Autodesk Inventor part; units mm, degrees
ref_plane "Work Plane1" through (0, 42.672, 0) normal (0, 1, 0) x (1, 0, 0)
ref_plane "YZ Plane" through (0, 0, 0) normal (1, 0, 0) x (0, 1, 0)
ref_plane "XZ Plane" through (0, 0, 0) normal (0, 1, 0) x (-1, 0, 0)
sketch "Sketch1" plane through (0, 0, 0) normal (0, 1, 0) x (-1, 0, 0)
  line L0 (-11.1125, 29.21) -> (11.1125, 29.21)
  line L1 (14.2875, 26.035) -> (14.2875, -26.035)
  line L2 (11.1125, -29.21) -> (-11.1125, -29.21)
  line L3 (-14.2875, -26.035) -> (-14.2875, 26.035)
  line L4 (-14.2875, 29.21) -> (14.2875, -29.21) construction
  line L5 (14.2875, 29.21) -> (-14.2875, -29.21) construction
  arc A0 (14.2875, 26.035) -> (11.1125, 29.21) centre (11.1125, 26.035) ccw
  arc A1 (-11.1125, 29.21) -> (-14.2875, 26.035) centre (-11.1125, 26.035) ccw
  arc A2 (-14.2875, -26.035) -> (-11.1125, -29.21) centre (-11.1125, -26.035) ccw
  arc A3 (11.1125, -29.21) -> (14.2875, -26.035) centre (11.1125, -26.035) ccw
  point P0 (0, 0)
  dimension "d0" = 28.575
  dimension "d1" = 58.42
  dimension "d2" = 3.175
extrude "Extrusion1" add sketch "Sketch1" along normal blind 46.482
ref_plane "Work Plane1" through (0, 42.672, 0) normal (0, 1, 0) x (1, 0, 0)
sketch "Sketch2" plane through (0, 42.672, 0) normal (0, 1, 0) x (1, 0, 0)
  arc A0 (-11.1125, 29.21) -> (-14.2875, 26.035) centre (-11.1125, 26.035) ccw
  line L0 (-11.1125, 29.21) -> (11.1125, 29.21)
  arc A1 (14.2875, 26.035) -> (11.1125, 29.21) centre (11.1125, 26.035) ccw
  line L1 (14.2875, 26.035) -> (14.2875, -26.035)
  arc A2 (11.1125, -29.21) -> (14.2875, -26.035) centre (11.1125, -26.035) ccw
  line L2 (11.1125, -29.21) -> (-11.1125, -29.21)
  arc A3 (-14.2875, -26.035) -> (-11.1125, -29.21) centre (-11.1125, -26.035) ccw
  line L3 (-14.2875, -26.035) -> (-14.2875, 26.035)
  line L4 (-11.1125, -36.8935) -> (11.1125, -36.8935)
  line L5 (14.2875, -33.7185) -> (14.2875, 33.7185)
  line L6 (11.1125, 36.8935) -> (-6.604, 36.8935)
  line L7 (-14.2875, 33.7185) -> (-14.2875, -33.7185)
  line L8 (-14.2875, -36.8935) -> (14.2875, 36.8935) construction
  line L9 (14.2875, -36.8935) -> (-14.2875, 36.8935) construction
  arc A4 (-11.1125, 36.8935) -> (-14.2875, 33.7185) centre (-11.1125, 33.7185) ccw
  arc A5 (14.2875, 33.7185) -> (11.1125, 36.8935) centre (11.1125, 33.7185) ccw
  arc A6 (11.1125, -36.8935) -> (14.2875, -33.7185) centre (11.1125, -33.7185) ccw
  arc A7 (-14.2875, -33.7185) -> (-11.1125, -36.8935) centre (-11.1125, -33.7185) ccw
  line L10 (-7.874, -33.655) -> (7.874, -33.655) construction
  line L11 (7.874, -33.655) -> (7.874, 33.655) construction
  line L12 (7.874, 33.655) -> (-7.874, 33.655) construction
  line L13 (-7.874, 33.655) -> (-7.874, -33.655) construction
  line L14 (-7.874, -33.655) -> (7.874, 33.655) construction
  line L15 (7.874, -33.655) -> (-7.874, 33.655) construction
  arc A8 (-9.144, 35.0749) -> (-6.604, 35.0749) centre (-7.874, 33.655) ccw
  line L16 (-9.144, 32.385) -> (-6.604, 32.385) construction
  line L17 (-6.604, 32.385) -> (-6.604, 34.925) construction
  line L18 (-6.604, 34.925) -> (-9.144, 34.925) construction
  line L19 (-9.144, 34.925) -> (-9.144, 32.385) construction
  line L20 (-9.144, 32.385) -> (-6.604, 34.925) construction
  line L21 (-6.604, 32.385) -> (-9.144, 34.925) construction
  line L22 (-9.144, 34.925) -> (-6.604, 34.925) construction
  line L23 (-6.604, 34.925) -> (-6.604, 36.8935)
  line L24 (-6.604, 36.8935) -> (-9.144, 36.8935)
  line L25 (-9.144, 36.8935) -> (-9.144, 34.925)
  arc A9 (-6.604, 35.0749) -> (-9.144, 35.0749) centre (-7.874, 33.655) ccw construction
  line L26 (-9.144, 36.8935) -> (-11.1125, 36.8935)
  line L27 (-6.604, 36.8935) -> (-9.144, 36.8935) construction
  arc A10 (6.604, 35.0749) -> (9.144, 35.0749) centre (7.874, 33.655) ccw
  line L28 (6.604, 36.8935) -> (6.604, 34.925)
  line L29 (9.144, 34.925) -> (9.144, 36.8935)
  line L30 (-14.2875, 0) -> (14.2875, 0) construction
  arc A11 (-6.604, -35.0749) -> (-9.144, -35.0749) centre (-7.874, -33.655) ccw
  line L31 (-6.604, -34.925) -> (-6.604, -36.8935)
  line L32 (-9.144, -36.8935) -> (-9.144, -34.925)
  arc A12 (9.144, -35.0749) -> (6.604, -35.0749) centre (7.874, -33.655) ccw
  line L33 (6.604, -36.8935) -> (6.604, -34.925)
  line L34 (9.144, -34.925) -> (9.144, -36.8935)
  line L35 (6.604, 36.8935) -> (9.144, 36.8935) construction
  line L36 (6.604, -36.8935) -> (9.144, -36.8935) construction
  line L37 (-9.144, -36.8935) -> (-6.604, -36.8935) construction
  line L38 (6.604, 36.8935) -> (9.144, 36.8935)
  line L39 (6.604, -36.8935) -> (9.144, -36.8935)
  line L40 (-9.144, -36.8935) -> (-6.604, -36.8935)
  point P0 (0, 0)
  dimension "d6" = 73.787
  dimension "d7" = 3.175
  dimension "d10" = 15.748
  dimension "d11" = 67.31
  dimension "d12" = 3.81
  dimension "d16" = 2.54
  dimension "d17" = 2.54
  dimension "d20" = 15.748
extrude "Extrusion2" add sketch "Sketch2" against normal blind 3.81 contours A0 L7 A4 L26 L25 A8 L23 L6 L28 A10 L29 A5 L5 A1 L0 | A3 L2 A2 L5 A6 L4 L34 A12 L33 L31 A11 L32 A7 L7 | L24 L23 A8 L25 | L32 A11 L31 L4 | L29 A10 L28 L6 | L4 L33 A12 L34
extrude "Extrusion3" cut sketch "Sketch2" against normal through all contours L24 L23 A8 L25 | L32 A11 L31 L4 | L29 A10 L28 L6 | L4 L33 A12 L34
sketch "Sketch3" plane through (0, 46.482, 0) normal (0, 1, 0) x (1, 0, 0)
  line L0 (-14.2875, 26.035) -> (-14.2875, -26.035) construction
  arc A0 (-14.2875, -26.035) -> (-11.1125, -29.21) centre (-11.1125, -26.035) ccw construction
  line L1 (-11.1125, -29.21) -> (11.1125, -29.21) construction
  arc A1 (11.1125, -29.21) -> (14.2875, -26.035) centre (11.1125, -26.035) ccw construction
  line L2 (14.2875, -26.035) -> (14.2875, 26.035) construction
  arc A2 (14.2875, 26.035) -> (11.1125, 29.21) centre (11.1125, 26.035) ccw construction
  line L3 (11.1125, 29.21) -> (-11.1125, 29.21) construction
  arc A3 (-11.1125, 29.21) -> (-14.2875, 26.035) centre (-11.1125, 26.035) ccw construction
  circle A4 centre (0, 14.9225) radius 14.2875
  line L4 (-13.3985, -18.034) -> (-13.3985, 9.9614)
  line L5 (13.3985, -18.034) -> (13.3985, 9.9614)
  line L6 (-13.3985, -18.034) -> (13.3985, -18.034)
  circle A5 centre (0, -18.034) radius 6.35 construction
  line L7 (0, -18.034) -> (0, -21.844) construction
  arc A6 (-6.35, -18.034) -> (6.35, -18.034) centre (0, -14.6473) ccw
  point P0 (0, 0)
  dimension "d27" = 0.889
  dimension "d28" = 0.889
  dimension "d29" = 47.244
  dimension "d30" = 12.7
  dimension "d31" = 3.81
extrude "Extrusion4" add sketch "Sketch3" along normal blind 3.81
sketch "Sketch4" plane through (0, 50.292, 0) normal (0, 1, 0) x (1, 0, 0)
  arc A0 (13.3985, 9.9614) -> (-13.3985, 9.9614) centre (0, 14.9225) ccw construction
  circle A1 centre (0, 14.9225) radius 6.9215
  point P0 (0, 0)
  dimension "d34" = 13.843
extrude "Extrusion5" add sketch "Sketch4" along normal blind 2.54
sketch "Sketch5" plane through (0, 50.292, 0) normal (0, 1, 0) x (1, 0, 0)
  circle A0 centre (0, 14.9225) radius 6.9215 construction
  arc A1 (-6.35, -18.034) -> (6.35, -18.034) centre (0, -14.6473) ccw construction
  line L0 (6.35, -18.034) -> (13.3985, -18.034) construction
  line L1 (13.3985, -18.034) -> (13.3985, 9.9614) construction
  arc A2 (13.3985, 9.9614) -> (-13.3985, 9.9614) centre (0, 14.9225) ccw construction
  line L2 (-13.3985, 9.9614) -> (-13.3985, -18.034) construction
  line L3 (-13.3985, -18.034) -> (-6.35, -18.034) construction
  line L4 (-9.906, -2.159) -> (9.9036, -2.159) construction
  line L5 (9.9036, -2.159) -> (9.9036, -14.859) construction
  line L6 (9.9036, -14.859) -> (-9.906, -14.859) construction
  line L7 (-9.906, -14.859) -> (-9.906, -2.159) construction
  point P0 (0, 0)
  dimension "d53" = 12.7
  dimension "d59" = 3.175
  dimension "d60" = 3.4925
  dimension "d61" = 3.4949
decal "Decal1"
sketch "Sketch6" plane through (0, 52.832, -14.9225) normal (0, 1, 0) x (1, 0, 0)
  circle A0 centre (0, 0) radius 6.9215 construction
  circle A1 centre (0, 0) radius 2.8575
  point P0 (0, -14.9225)
  dimension "d62" = 5.715
extrude "Extrusion6" add sketch "Sketch6" along normal blind 3.175
hole "Hole1" at (0, 56.007, -14.9225) direction (0, -1, 0) diameter 2.54 depth 25.4 tip angle 118 countersink diameter 3.81 countersink angle 82
sketch "Sketch7" plane through (0, 0, 0) normal (0, -1, 0) x (1, 0, 0)
  line L0 (-14.2875, 26.035) -> (-14.2875, -26.035) construction
  arc A0 (-14.2875, -26.035) -> (-11.1125, -29.21) centre (-11.1125, -26.035) ccw construction
  line L1 (-11.1125, -29.21) -> (11.1125, -29.21) construction
  arc A1 (11.1125, -29.21) -> (14.2875, -26.035) centre (11.1125, -26.035) ccw construction
  line L2 (14.2875, -26.035) -> (14.2875, 26.035) construction
  arc A2 (14.2875, 26.035) -> (11.1125, 29.21) centre (11.1125, 26.035) ccw construction
  line L3 (11.1125, 29.21) -> (-11.1125, 29.21) construction
  arc A3 (-11.1125, 29.21) -> (-14.2875, 26.035) centre (-11.1125, 26.035) ccw construction
  line L4 (-14.2875, 26.035) -> (-14.2875, 33.7185) construction
  line L5 (14.2875, -26.035) -> (14.2875, -33.7185) construction
  line L6 (-14.2875, 29.21) -> (14.2875, 29.21) construction
  line L7 (14.2875, 29.21) -> (14.2875, -29.21) construction
  line L8 (14.2875, -29.21) -> (-14.2875, -29.21) construction
  line L9 (-14.2875, -29.21) -> (-14.2875, 29.21) construction
  line L10 (-11.1125, 22.86) -> (-14.2875, 22.86)
  line L11 (-14.2875, 22.86) -> (-14.2875, 29.21)
  line L12 (-14.2875, 29.21) -> (-7.9375, 29.21)
  line L13 (-7.9375, 29.21) -> (-7.9375, 26.035)
  line L14 (-7.9375, 22.86) -> (-14.2875, 29.21) construction
  line L15 (-14.2875, 22.86) -> (-7.9375, 29.21) construction
  line L16 (11.1125, 22.86) -> (14.2875, 22.86)
  line L17 (14.2875, 22.86) -> (14.2875, 29.21)
  line L18 (14.2875, 29.21) -> (7.9375, 29.21)
  line L19 (7.9375, 29.21) -> (7.9375, 26.035)
  line L20 (7.9375, 22.86) -> (14.2875, 29.21) construction
  line L21 (14.2875, 22.86) -> (7.9375, 29.21) construction
  line L22 (-11.1125, -22.86) -> (-14.2875, -22.86)
  line L23 (-14.2875, -22.86) -> (-14.2875, -29.21)
  line L24 (-14.2875, -29.21) -> (-7.9375, -29.21)
  line L25 (-7.9375, -29.21) -> (-7.9375, -26.035)
  line L26 (-7.9375, -22.86) -> (-14.2875, -29.21) construction
  line L27 (-14.2875, -22.86) -> (-7.9375, -29.21) construction
  line L28 (11.1125, -22.86) -> (14.2875, -22.86)
  line L29 (14.2875, -22.86) -> (14.2875, -29.21)
  line L30 (14.2875, -29.21) -> (7.9375, -29.21)
  line L31 (7.9375, -29.21) -> (7.9375, -26.035)
  line L32 (7.9375, -22.86) -> (14.2875, -29.21) construction
  line L33 (14.2875, -22.86) -> (7.9375, -29.21) construction
  arc A4 (-11.1125, 22.86) -> (-7.9375, 26.035) centre (-11.1125, 26.035) ccw
  arc A5 (7.9375, 26.035) -> (11.1125, 22.86) centre (11.1125, 26.035) ccw
  arc A6 (-7.9375, -26.035) -> (-11.1125, -22.86) centre (-11.1125, -26.035) ccw
  arc A7 (11.1125, -22.86) -> (7.9375, -26.035) centre (11.1125, -26.035) ccw
  point P0 (0, 0)
  dimension "d76" = 3.175
extrude "Extrusion7" cut sketch "Sketch7" against normal blind 1.27
properties part number "HS-785HB-1111-2017" material "Plastic, Opaque Black"
For this review, take the finished solid that the model builds, in its own axes (mm). A direction names the side the tool comes from. Give positions to 0.01 mm unless a question says otherwise; leave off trailing zeros. Loops run counter-clockwise (first coordinate to the right, second up) from the corner with the lowest first, then second, coordinate; pieces in that order, holes last.
Item 1: Draft analysis for pull direction Z (two halves, no side actions). For faces 1 (the cylindrical face through (-7.94, 40.79, -31.75)), 2 (the cylindrical face through (3.194, 51.544, -21.063)), 3 (the flat face through (-9.144, 41, 36)), state which applies: +Z half, -Z half, draft (parallel to the pull), parting line (faces both ways), or undercut.
Item 2: Take a section at C-C, the plane z = -3. State the section outline as (x, y) points.
Item 3: Insertion check: pin 1 (2 mm diameter, centred on y = 41.5, z = 36, fed in from +X); pin 2 (12 mm diameter, centred on x = 4, y = 27.5, fed in from -Z); pin 3 (5 mm diameter, centred on y = 49.5, z = -28.5, fed in from -X); pin 4 (2.5 mm diameter, centred on x = 0, z = -14.92, fed in from -Y). Each pin has a flat end and moves straight along its axis. Give the tip position at first contact, or say it passes through.
Item 4: Take a section at D-D, the plane x = -12. State the section outline as (y, z) points.
Item 5: For line 1 along Z through (x, y) = (0, 38.75); line 2 along Z through (x, y) = (-4.75, 45.5); line 3 along Y through (x, z) = (13, -21.5), list the stretches that pass through material, from the lowest coordinate up.
Item 6: Tool access review of faces 4 (the flat face through (0, 19, -29.21)), 5 (the cylindrical face through (0.49, 42.77, -13.75)), 6 (the cylindrical face through (-13.38, 19.8, -28.26)), 7 (the flat face through (6.604, 41, -36)), 8 (the flat face through (13.398, 48, 4)): name each direction out of +Z, -Z, +X, -X, +Y, -Y from which nothing blocks a thin tool from reaching the whole face with its end or side.
Calculated:
1. face 1: undercut
1. face 2: parting line
1. face 3: draft
2. outline: (-14.29, 0) - (14.29, 0) - (14.29, 46.48) - (13.4, 46.48) - (13.4, 50.29) - (-13.4, 50.29) - (-13.4, 46.48) - (-14.29, 46.48) - close
3. pin 1: stops at x = 14.02
3. pin 2: stops at z = -29.21
3. pin 3: stops at x = -9.02
3. pin 4: stops at y = 0
4. outline: (0, -22.86) - (1.27, -22.86) - (1.27, -29.08) - (38.86, -29.08) - (38.86, -36.77) - (42.67, -36.77) - (42.67, -29.08) - (46.48, -29.08) - (46.48, -22.68) - (50.29, -22.68) - (50.29, 18.03) - (46.48, 18.03) - (46.48, 29.08) - (42.67, 29.08) - (42.67, 36.77) - (38.86, 36.77) - (38.86, 29.08) - (1.27, 29.08) - (1.27, 22.86) - (0, 22.86) - close
5. line 1: z = -29.21 to -16.19, -13.65 to 29.21
5. line 2: z = -29.21 to 29.21
5. line 3: y = 0 to 46.48
6. face 4: -Z, +X, -X, -Y
6. face 5: +Y
6. face 6: -Z, -X, -Y
6. face 7: -Z, +Y, -Y
6. face 8: +Z, +X, +Y
